Could you check a few things on this model? Use its own coordinates, in mm. Face numbers are marked on the shaded views. Give positions to 0.01 mm unless a question says otherwise; leave off trailing zeros. Loops run counter-clockwise (first coordinate to the right, second up) from the corner with the lowest first, then second, coordinate; pieces in that order, holes last. Notation, with made-up numbers: M -3,57.25 L 48,57.25 A27 cw 48,94.25 Z; hole C 53,15 d8. An arc over 180 degrees is marked long. Answer in a Markdown table with one row per item. Add a question column.
1. If we section it at A-A on x = 0: List the corners of the cut face in (y, z) for me, then the cut area to 3 significant figures.
2. Thinking about a two-plate mould opening in X: for the marked faces 1 and 2, which applies, released by +X, released by -X, zero draft, split by the parting line, or undercut?
3. I need wall thicknesses on line 1 along Z through (x, y) = (0, 5.7); line 2 along Y through (x, z) = (0, 1); line 3 along X through (y, z) = (0.25, 7.25). Which ranges of each line are inside material? Lowest first, please. Write a range as from..to.
4. If we section it at B-B on y = 0: List the corners of the cut face in (x, z) for me.
5. I'm going to push a flat-ended pin straight in: pin 1 Ø5.5 at (x, z) = (0, 5) entering from -Y. Where does the tip first touch, or does it pass through?
6. If we section it at D-D on z = 13: List the corners of the cut face in (x, y) for me.
7. If we section it at C-C on z = 5: List the corners of the cut face in (x, y) for me.
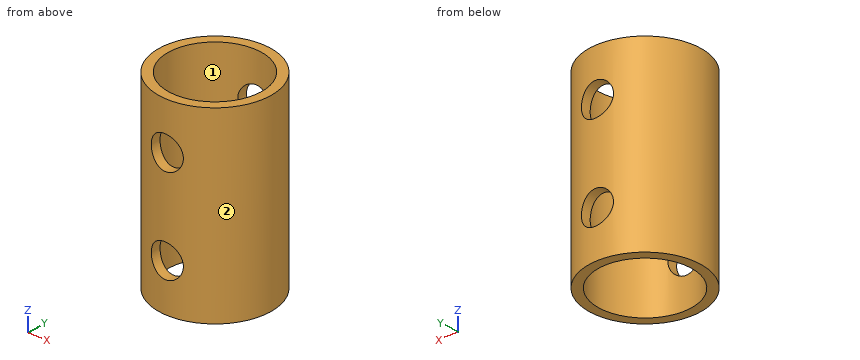
Autodesk Inventor part; units mm, degrees
ref_plane "YZ Plane" through (0, 0, 0) normal (1, 0, 0) x (0, 1, 0)
ref_plane "XZ Plane" through (0, 0, 0) normal (0, 1, 0) x (-1, 0, 0)
ref_plane "XY Plane" through (0, 0, 0) normal (0, 0, 1) x (1, 0, 0)
sketch "Sketch1" plane through (0, 0, 0) normal (0, 0, 1) x (1, 0, 0)
  point P0 (0, 0)
sketch "Sketch2" plane through (0, 0, 0) normal (0, 0, 1) x (1, 0, 0)
  circle A0 centre (0, 0) radius 6
  dimension "d0" = 12
extrude "Extrusion1" add sketch "Sketch2" along normal blind 20
sketch "Sketch3" plane through (0, 0, 0) normal (1, 0, 0) x (0, 1, 0)
  point P0 (0, 0)
sketch "Sketch4" plane through (0, 0, 20) normal (0, 0, 1) x (1, 0, 0)
  circle A0 centre (0, 0) radius 5
  dimension "d3" = 10
extrude "Extrusion2" cut sketch "Sketch4" against normal through all
sketch "Sketch5" plane through (0, 0, 0) normal (0, 1, 0) x (-1, 0, 0)
  line L0 (6, 20) -> (-6, 20)
  line L1 (0, 20) -> (0, 15)
  line L2 (0, 15) -> (0, 5)
  circle A0 centre (0, 15) radius 1.75
  circle A1 centre (0, 5) radius 1.75
  point P0 (0, 0)
  dimension "d6" = 5
  dimension "d7" = 10
  dimension "d8" = 3.5
  dimension "d9" = 3.5
extrude "Extrusion3" cut sketch "Sketch5" along normal through all both and the other way through all
properties part number "two way connector for capping system"
Results:
| question | item | result |
|---|---|---|
| 1 | outline | M -6,0 L -5,0 L -5,3.25 L -6,3.25 Z; M -6,6.75 L -5,6.75 L -5,13.25 L -6,13.25 Z; M -6,16.75 L -5,16.75 L -5,20 L -6,20 Z; M 5,0 L 6,0 L 6,3.25 L 5,3.25 Z; M 5,6.75 L 6,6.75 L 6,13.25 L 5,13.25 Z; M 5,16.75 L 6,16.75 L 6,20 L 5,20 Z |
| 1 | area | 26.0 mm2 |
| 2 | face 1 | undercut |
| 2 | face 2 | split by the parting line |
| 3 | line 1 | 0..3.25, 6.75..13.25, 16.75..20 |
| 3 | line 2 | -6..-5, 5..6 |
| 3 | line 3 | -5.99..-4.99, 4.99..5.99 |
| 4 | outline | M -6,0 L -5,0 L -5,20 L -6,20 Z; M 5,0 L 6,0 L 6,20 L 5,20 Z |
| 5 | pin 1 | y = -6 |
| 6 | outline | C 0,0 d12; hole C 0,0 d10 |
| 7 | outline | M -1.75,-5.74 L -1.75,-4.68 A5 cw -1.75,4.68 L -1.75,5.74 A6 ccw Z; M 1.75,-5.74 A6 ccw 1.75,5.74 L 1.75,4.68 A5 cw 1.75,-4.68 Z |
